Can you work these out from the model? Positions are in its coordinate system, mm. Face numbers are marked on the shaded views. Coordinates: 2 decimals unless noted, no trailing zeros. Write each loop counter-clockwise with the first axis right and the second up, starting at its lowest first coordinate (ties: lowest second). Pieces come first, ordered by that corner, then holes. Notation, with made-up numbers: (-30.75, 17) -> (-2.75, 17) arc R19 cw to (-2.75, 35) -> close; hole circle Ø7 at (38.25, -1). An arc over 180 degrees is marked (long way). Use one line per item in the form item = value.
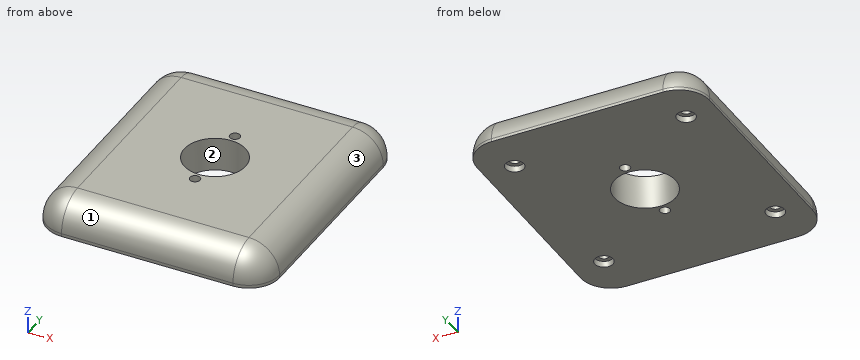
```python
from build123d import *

# Parameters (mm, degrees)
CROQUIS1_W              = 76
CROQUIS1_H              = 85
SALIENTE_EXTRUIR1_DEPTH = 11
CROQUIS3_R              = 1.65
CORTAR_EXTRUIR2_DEPTH   = 5
CROQUIS4_R              = 3
CORTAR_EXTRUIR3_DEPTH   = 2
REDONDEO3_R             = 10
CROQUIS5_R              = 10
CROQUIS5_R_2            = 1.65
CORTAR_EXTRUIR4_DEPTH   = 12


with BuildPart() as part:
    # Croquis1 → Saliente-Extruir1 (new body)
    with BuildSketch(Plane.XY):
        Rectangle(CROQUIS1_W, CROQUIS1_H)
    extrude(amount=SALIENTE_EXTRUIR1_DEPTH)

    # Croquis3 → Cortar-Extruir2 (cut)
    with BuildSketch(Plane(origin=(0, 0, 0), x_dir=(-1, 0, 0), z_dir=(0, 0, -1))):
        with Locations((28, -28)):
            Circle(CROQUIS3_R)
        with Locations((-28, -28)):
            Circle(CROQUIS3_R)
        with Locations((-28, 28)):
            Circle(CROQUIS3_R)
        with Locations((28, 28)):
            Circle(CROQUIS3_R)
    extrude(amount=-CORTAR_EXTRUIR2_DEPTH, mode=Mode.SUBTRACT)

    # Croquis4 → Cortar-Extruir3 (cut)
    with BuildSketch(Plane(origin=(0, 0, 0), x_dir=(-1, 0, 0), z_dir=(0, 0, -1))):
        with Locations((28, 28)):
            Circle(CROQUIS4_R)
        with Locations((28, -28)):
            Circle(CROQUIS4_R)
        with Locations((-28, 28)):
            Circle(CROQUIS4_R)
        with Locations((-28, -28)):
            Circle(CROQUIS4_R)
    extrude(amount=-CORTAR_EXTRUIR3_DEPTH, mode=Mode.SUBTRACT)

    # Redondeo3
    redondeo3_edges = [part.edges().sort_by_distance(p)[0] for p in [
        (38, 0, 11),
        (0, 42.5, 11),
        (-38, 0, 11),
        (0, -42.5, 11),
        (-38, 42.5, 5.5),
        (38, 42.5, 5.5),
        (38, -42.5, 5.5),
        (-38, -42.5, 5.5),
    ]]
    fillet(redondeo3_edges, radius=REDONDEO3_R)

    # Croquis5 → Cortar-Extruir4 (cut, through all)
    with BuildSketch(Plane(origin=(0, 0, 0), x_dir=(-1, 0, 0), z_dir=(0, 0, -1))):
        Circle(CROQUIS5_R)
        with Locations((0, 12.5)):
            Circle(CROQUIS5_R_2)
        with Locations((0, -12.5)):
            Circle(CROQUIS5_R_2)
    extrude(amount=-CORTAR_EXTRUIR4_DEPTH, mode=Mode.SUBTRACT)


solid = part.part
```
Q1. Suppose I cut it at B-B (z = 10). Write out the boundary of the cut face in (x, y).
Return value:
outline = (-32.36, -32.5) arc R4.36 ccw to (-28, -36.86) -> (28, -36.86) arc R4.36 ccw to (32.36, -32.5) -> (32.36, 32.5) arc R4.36 ccw to (28, 36.86) -> (-28, 36.86) arc R4.36 ccw to (-32.36, 32.5) -> close; hole circle Ø20 at (0, 0); hole circle Ø3.3 at (0, -12.5); hole circle Ø3.3 at (0, 12.5)
Q2. Suppose I cut it at C-C (y = 28). Write out the boundary of the cut face in (x, z).
Return value:
outline = (-38, 0) -> (-31, 0) -> (-31, 2) -> (-29.65, 2) -> (-29.65, 5) -> (-26.35, 5) -> (-26.35, 2) -> (-25, 2) -> (-25, 0) -> (25, 0) -> (25, 2) -> (26.35, 2) -> (26.35, 5) -> (29.65, 5) -> (29.65, 2) -> (31, 2) -> (31, 0) -> (38, 0) -> (38, 1) arc R10 ccw to (28, 11) -> (-28, 11) arc R10 ccw to (-38, 1) -> close
Q3. Suppose I cut it at D-D (y = 0). Write out the boundary of the cut face in (x, z), then the cut area to 3 significant figures.
Return value:
outline = (-38, 0) -> (-10, 0) -> (-10, 11) -> (-28, 11) arc R10 ccw to (-38, 1) -> close; (10, 0) -> (38, 0) -> (38, 1) arc R10 ccw to (28, 11) -> (10, 11) -> close
area = 573 mm2
Q4. Will these pins go through, and if not, where does the flat tip stop? pin 1 (4 mm diameter, centred on x = 28, y = 28, fed in from -Z); pin 2 (1.6 mm diameter, centred on x = -27.5, y = -28.5, fed in from -Z); pin 3 (1 mm diameter, centred on x = -3, z = 4, fed in from -Y).
Return value:
pin_1 = 2
pin_2 = 5
pin_3 = -42.18
Q5. If I drill on line 1 (Y direction, x = 28, z = 2.8); line 2 (Y direction, x = 0, z = 7.5); line 3 (Y direction, x = 0, z = 3.25), over which ranges is the centre line in solid material (lowest first)? Write a range as from..to.
Return value:
line_1 = -42.34..-29.65, -26.35..26.35, 29.65..42.34
line_2 = -40.1..-14.15, -10.85..-10, 10..10.85, 14.15..40.1
line_3 = -42.24..-14.15, -10.85..-10, 10..10.85, 14.15..42.24
Q6. Suppose I cut it at A-A (y = 12.5). Write out the boundary of the cut face in (x, z).
Return value:
outline = (-38, 0) -> (-1.65, 0) -> (-1.65, 11) -> (-28, 11) arc R10 ccw to (-38, 1) -> close; (1.65, 0) -> (38, 0) -> (38, 1) arc R10 ccw to (28, 11) -> (1.65, 11) -> close
Q7. Thinking about a two-plate mould opening in X: for the marked faces 1, 2 and 3, which applies, released by +X, released by -X, zero draft, split by the parting line, or undercut?
Return value:
face_1 = zero draft
face_2 = undercut
face_3 = released by +X
